```python
from build123d import *

# Parameters (mm, degrees)
F1_DEPTH = 4
F2_R     = 5
F3_R     = 1
F4_SIZE  = 0.5


with BuildPart() as f1:
    # F0 (on Top) → F1 (new body)
    with BuildSketch(Plane.XY):
        with BuildLine():
            ThreePointArc((0, 3), (2.802517, 1.070466), (2, -2.236068))
            Line((2, -2.236068), (2, -7.228416))
            ThreePointArc((2, -7.228416), (2.678825, -7.005276), (3.333333, -6.718548))
            ThreePointArc((3.333333, -6.718548), (10, -5.155644), (16.666667, -6.718548))
            ThreePointArc((16.666667, -6.718548), (17.321175, -7.005276), (18, -7.228416))
            Line((18, -7.228416), (18, -2.236068))
            ThreePointArc((18, -2.236068), (20, 3), (22, -2.236068))
            Line((22, -2.236068), (22, -7.228416))
            ThreePointArc((22, -7.228416), (27.005276, 2.678825), (16.666667, 6.718548))
            ThreePointArc((16.666667, 6.718548), (10, 5.155644), (3.333333, 6.718548))
            ThreePointArc((3.333333, 6.718548), (1.711854, 7.302024), (0, 7.5))
            Line((0, 7.5), (-39, 7.5))
            ThreePointArc((-39, 7.5), (-46.5, 0), (-39, -7.5))
            Line((-39, -7.5), (-2, -7.5))
            Line((-2, -7.5), (-2, -3))
            Line((-2, -3), (-39, -3))
            ThreePointArc((-39, -3), (-42, 0), (-39, 3))
            Line((-39, 3), (0, 3))
        make_face()
    extrude(amount=F1_DEPTH)

    # F2
    f2_edges = [f1.edges().sort_by_distance(p)[0] for p in [
        (2, -2.236068, 2),
        (18, -2.236068, 2),
        (22, -2.236068, 2),
    ]]
    fillet(f2_edges, radius=F2_R)

    # F3
    f3_edges = [f1.edges().sort_by_distance(p)[0] for p in [
        (-2, -3, 2),
        (2, -7.228416, 2),
        (-2, -7.5, 2),
        (18, -7.228416, 2),
        (22, -7.228416, 2),
    ]]
    fillet(f3_edges, radius=F3_R)

    # F4
    f4_edges = [f1.edges().sort_by_distance(p)[0] for p in [
        (-21, -7.5, 4),
        (-21, -7.5, 0),
    ]]
    chamfer(f4_edges, length=F4_SIZE)


solid = f1.part
```
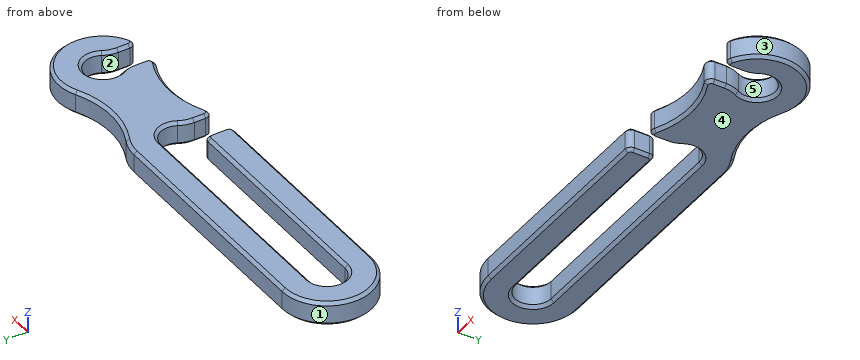
Verification items for the finished model (mm, model axes). Face numbers are marked on the shaded views. A direction names the side the tool comes from. Coordinates: 2 decimals unless noted, no trailing zeros. Loops run counter-clockwise (first coordinate to the right, second up) from the corner with the lowest first, then second, coordinate; pieces in that order, holes last. Notation, with made-up numbers: (-17, 68) - (-1, 68) arc R29 cw to (-1, 101) - close; hole circle Ø2 at (-23, 37.5). An arc over 180 degrees is marked (long way). Return JSON: item names as keys, results as strings.
1. Go/stop test with flat-tipped pins: pin 1 (2 mm diameter, centred on y = -5, z = 2.5, fed in from +X); pin 2 (0.9 mm diameter, centred on y = -5, z = 2, fed in from -X); pin 3 (1.5 mm diameter, centred on y = -4.5, z = 2.5, fed in from -X). Record where each tip stops, or that it passes through.
Established:
{"pin 1": "stops at x = 26.34", "pin 2": "stops at x = -44.96", "pin 3": "stops at x = -45.5"}
2. Section check A-A, the plane y = 0. Record the boundary of the cut face in (x, z).
Established:
{"outline": "(-46.5, 0.5) - (-46, 0) - (-42.5, 0) - (-42, 0.5) - (-42, 3.5) - (-42.5, 4) - (-46, 4) - (-46.5, 3.5) - close; (3, 0.5) - (3.5, 0) - (16.5, 0) - (17, 0.5) - (17, 3.5) - (16.5, 4) - (3.5, 4) - (3, 3.5) - close; (23, 0.5) - (23.5, 0) - (27, 0) - (27.5, 0.5) - (27.5, 3.5) - (27, 4) - (23.5, 4) - (23, 3.5) - close"}
3. Section check C-C, the plane x = 20. Record the boundary of the cut face in (y, z), then the cut area to 3 significant figures.
Established:
{"outline": "(3, 0.5) - (3.5, 0) - (7, 0) - (7.5, 0.5) - (7.5, 3.5) - (7, 4) - (3.5, 4) - (3, 3.5) - close", "area": "17.5 mm2"}
4. Thickness scan on L1, parallel to X at y = 0, z = 2.15; L2, parallel to X at y = -1.25, z = 3.6; L3, parallel to Y at x = -10, z = 1.05. Record the ranges inside material, lowest first.
Established:
{"L1": "x = -46.5 to -42, 3 to 17, 23 to 27.5", "L2": "x = -46.29 to -41.84, 2.84 to 17.16, 22.84 to 27.29", "L3": "y = -7.5 to -3, 3 to 7.5"}
5. Section check B-B, the plane x = -12. Record the boundary of the cut face in (y, z).
Established:
{"outline": "(-7.5, 0.5) - (-7, 0) - (-3.5, 0) - (-3, 0.5) - (-3, 3.5) - (-3.5, 4) - (-7, 4) - (-7.5, 3.5) - close; (3, 0.5) - (3.5, 0) - (7, 0) - (7.5, 0.5) - (7.5, 3.5) - (7, 4) - (3.5, 4) - (3, 3.5) - close"}
6. Mould release check, pull along Y, two halves, no side actions. Record for the marked faces 3, 4 and 5: +Y half, -Y half, draft (parallel to the pull), parting line (faces both ways), or undercut.
Established:
{"face 3": "parting line", "face 4": "draft", "face 5": "undercut"}
7. Tool access check on the marked faces 1 and 2. Record the directions out of +Z, -Z, +X, -X, +Y, -Y that give a thin tool (end or side, any length) a straight path to the whole face; none if there is none.
Established:
{"face 1": "+Z, -Z, -X", "face 2": "+Z, -Z"}
